from build123d import *

# Parameters (mm, degrees)
F0_R     = 6.5
F1_DEPTH = 1.6
F3_DEPTH = 64
F4_R     = 4.5
F5_DEPTH = 7.5
F6_R     = 4.5


with BuildPart() as f1:
    # F0 (on Top) → F1 (new body)
    with BuildSketch(Plane.XY):
        Circle(F0_R)
    extrude(amount=F1_DEPTH)

    # F2 (on face) → F3 (join)
    with BuildSketch(Plane(origin=(0, 0, 0), x_dir=(1, 0, 0), z_dir=(0, 0, -1))):
        Polygon((0.5, 1), (0, 1), (-0.5, 1), (-0.5, 0.5), (-1, 0.5), (-1, 0), (-1, -0.5), (-0.5, -0.5), (-0.5, -1), (0, -1), (0.5, -1), (0.5, -0.5), (1, -0.5), (1, 0), (1, 0.5), (0.5, 0.5), align=None)
    extrude(amount=F3_DEPTH)

    # F4 (on face) → F5 (join)
    with BuildSketch(Plane(origin=(0, 0, -64), x_dir=(1, 0, 0), z_dir=(0, 0, -1))):
        Circle(F4_R)
        Polygon((-0.5, 1), (0.5, 1), (0.5, 0.5), (1, 0.5), (1, -0.5), (0.5, -0.5), (0.5, -1), (-0.5, -1), (-0.5, -0.5), (-1, -0.5), (-1, 0.5), (-0.5, 0.5), align=None, mode=Mode.SUBTRACT)
        Polygon((0.5, 0.5), (0.5, 1), (-0.5, 1), (-0.5, 0.5), (-1, 0.5), (-1, -0.5), (-0.5, -0.5), (-0.5, -1), (0.5, -1), (0.5, -0.5), (1, -0.5), (1, 0.5), align=None)
    extrude(amount=F5_DEPTH)

    # F6
    f6_edges = [f1.edges().sort_by_distance(p)[0] for p in [
        (-4.5, 0, -71.5),
    ]]
    fillet(f6_edges, radius=F6_R)


solid = f1.part
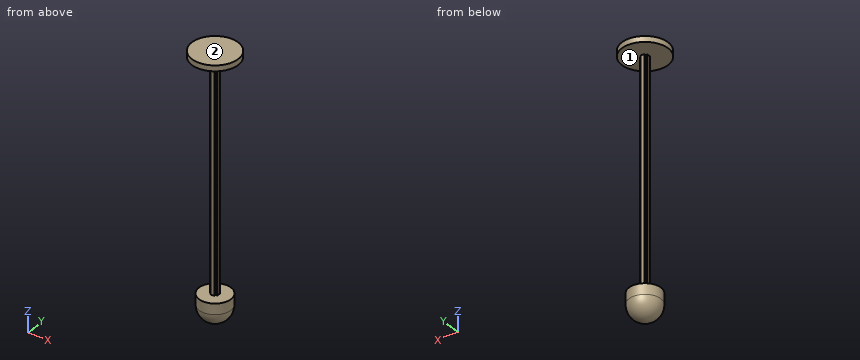
Source: CAD feature listing. Evaluate the final solid. Frame: model axes, mm. Face numbers are marked on the shaded views. Round coordinates to 2 decimals unless told otherwise and drop trailing zeros. Order: outer loops, then holes, each group sorted by start corner. A loop starts at its lowest first (then second) coordinate and runs counter-clockwise, first axis right, second up. Notation, with made-up numbers: (-23, 43.25) - (11, 43.25) arc R16 ccw to (11, 57.25) - close; hole circle Ø3 at (67, 13). An arc over 180 degrees is marked (long way). Use a Markdown table: item, result. Add a question column.
1. Section query B-B (z = -12.5). Return the cut outline in (x, y).
2. Mould query, pull axis Z, two halves, no side actions, for the marked faces 1 and 2. Classes: +Z half, -Z half, draft (parallel to the pull), parting line (faces both ways), or undercut.
3. Line query: probe 1 along Y at (x, z) = (0, -48); probe 2 along Z at (x, y) = (2.5, -4.75); probe 3 along Z at (x, y) = (3.5, 2). Output: solid intervals per line, ascending.
4. Section query A-A (y = -3.5). Return the cut outline in (x, z).
5. First-contact query: pin 1 (1.5 mm diameter, centred on y = 2, z = -17.5, fed in from +X); pin 2 (4 mm diameter, centred on y = 0.5, z = -56, fed in from -X); pin 3 (2 mm diameter, centred on x = 2.5, y = -2.5, fed in from -Z); pin 4 (0.6 mm diameter, centred on y = -0.5, z = -39, fed in from +X). Flat tips, straight axial feed; report the tip coordinate or a pass-through.
Derived:
| question | item | result |
|---|---|---|
| 1 | outline | (-1, -0.5) - (-0.5, -0.5) - (-0.5, -1) - (0.5, -1) - (0.5, -0.5) - (1, -0.5) - (1, 0.5) - (0.5, 0.5) - (0.5, 1) - (-0.5, 1) - (-0.5, 0.5) - (-1, 0.5) - close |
| 2 | face 1 | undercut |
| 2 | face 2 | +Z half |
| 3 | probe 1 | -1 to 1 |
| 3 | probe 2 | 0 to 1.6 |
| 3 | probe 3 | -69 to -64, 0 to 1.6 |
| 4 | outline | (-5.48, 0) - (5.48, 0) - (5.48, 1.6) - (-5.48, 1.6) - close; (-2.83, -67) arc R2.83 ccw to (2.83, -67) - (2.83, -64) - (-2.83, -64) - close |
| 5 | pin 1 | through |
| 5 | pin 2 | x = -1 |
| 5 | pin 3 | z = -70.72 |
| 5 | pin 4 | x = 1 |
